from build123d import *

# Parameters (mm, degrees)
SKETCH_1_R      = 3.5
EXTRUDE_1_DEPTH = 5
SKETCH_2_W      = 58
SKETCH_2_H      = 2
EXTRUDE_2_DEPTH = 4


with BuildPart() as part:
    # 草图1 → 凸台-拉伸1 (new body)
    with BuildSketch(Plane.XY):
        with BuildLine():
            Line((-7.608745595, -1.184004699), (-6, 7.5))
            Line((-6, 7.5), (6, 7.5))
            Line((6, 7.5), (7.608745595, -1.184004699))
            ThreePointArc((7.608745595, -1.184004699), (14, -6.5), (20.391254405, -1.184004699))
            Line((20.391254405, -1.184004699), (22, 7.5))
            Line((22, 7.5), (29, 7.5))
            Line((29, 7.5), (29, 11.5))
            Line((29, 11.5), (-29, 11.5))
            Line((-29, 11.5), (-29, 7.5))
            Line((-29, 7.5), (-22, 7.5))
            Line((-22, 7.5), (-20.391254405, -1.184004699))
            ThreePointArc((-20.391254405, -1.184004699), (-14, -6.5), (-7.608745595, -1.184004699))
        make_face()
        with Locations((-14, 0)):
            Circle(SKETCH_1_R, mode=Mode.SUBTRACT)
        with Locations((14, 0)):
            Circle(SKETCH_1_R, mode=Mode.SUBTRACT)
    extrude(amount=EXTRUDE_1_DEPTH)

    # 草图2 → 凸台-拉伸2 (add)
    with BuildSketch(Plane.XZ.offset(-7.5)):
        with Locations((0, 6)):
            Rectangle(SKETCH_2_W, SKETCH_2_H)
    extrude(amount=-EXTRUDE_2_DEPTH)


solid = part.part
Here's how the part is built. I have some questions about the finished solid (model axes, mm). A direction names the side the tool comes from. Coordinates: 2 decimals unless noted, no trailing zeros. Order: outer loops, then holes, each group sorted by start corner. A loop starts at its lowest first (then second) coordinate and runs counter-clockwise, first axis right, second up.
Item 1: If we section it at D-D on y = 5.25: List the corners of the cut face in (x, z) for me.
Result sheet:
outline: (-21.58, 0) - (-6.42, 0) - (-6.42, 5) - (-21.58, 5) - close; (6.42, 0) - (21.58, 0) - (21.58, 5) - (6.42, 5) - close
Item 2: For faces 4 (the face through (0, 7.5, 4)), 5 (the face through (-6.816, 3.097, 2.465)), 6 (the face through (14, 4, 5)), 7 (the face through (-29, 9, 3)), which set-ups out of +Z, -Z, +X, -X, +Y, -Y let a thin tool reach every point of the face, with its end or its side?
Result sheet:
face 4: +Z, -Y
face 5: +Z, -Z, -Y
face 6: +Z, +X, -X, -Y
face 7: +Z, -Z, -X, +Y, -Y
Item 3: If we section it at C-C on z = 2: List the corners of the cut face in (x, y) for me.
Result sheet:
outline: (-29, 7.5) - (-22, 7.5) - (-20.39, -1.18) arc R6.5 ccw to (-7.61, -1.18) - (-6, 7.5) - (6, 7.5) - (7.61, -1.18) arc R6.5 ccw to (20.39, -1.18) - (22, 7.5) - (29, 7.5) - (29, 11.5) - (-29, 11.5) - close; hole circle Ø7 at (-14, 0); hole circle Ø7 at (14, 0)
Item 4: For P1, Ø8, axis at x = 14, y = 0, coming from the -Z side; P2, Ø4, axis at x = 10.5, y = 4.5, coming from the +Z side, each with a flat end and sliding along its axis, tell me the tip position at first contact or that it passes through.
Result sheet:
P1: stops at z = 0
P2: stops at z = 5
Item 5: If we section it at B-B on y = 0: List the corners of the cut face in (x, z) for me.
Result sheet:
outline: (-20.61, 0) - (-17.5, 0) - (-17.5, 5) - (-20.61, 5) - close; (-10.5, 0) - (-7.39, 0) - (-7.39, 5) - (-10.5, 5) - close; (7.39, 0) - (10.5, 0) - (10.5, 5) - (7.39, 5) - close; (17.5, 0) - (20.61, 0) - (20.61, 5) - (17.5, 5) - close
Item 6: I need wall thicknesses on line 1 (Y direction, x = -14, z = 1.35); line 2 (X direction, y = -1.75, z = 1.25); line 3 (X direction, y = -3, z = 0.5). Which ranges of each line are inside material? Lowest first, please.
Result sheet:
line 1: y = -6.5 to -3.5, 3.5 to 11.5
line 2: x = -20.26 to -17.03, -10.97 to -7.74, 7.74 to 10.97, 17.03 to 20.26
line 3: x = -19.77 to -15.8, -12.2 to -8.23, 8.23 to 12.2, 15.8 to 19.77
Item 7: If we mould it in two halves opening along X, with no side actions, what happens to faces 1 (the face through (0, 9, 0)), 2 (the face through (21.184, 3.097, 2.465)), 3 (the face through (-10.66, 1.05, 2.46))? For each: +X half, -X half, draft (parallel to the pull), parting line (faces both ways), or undercut.
Result sheet:
face 1: draft
face 2: +X half
face 3: undercut
Item 8: If we section it at A-A on x = -14: List the corners of the cut face in (y, z) for me, plus the area to 3 significant figures.
Result sheet:
outline: (-6.5, 0) - (-3.5, 0) - (-3.5, 5) - (-6.5, 5) - close; (3.5, 0) - (11.5, 0) - (11.5, 7) - (7.5, 7) - (7.5, 5) - (3.5, 5) - close
area: 63.0 mm2
